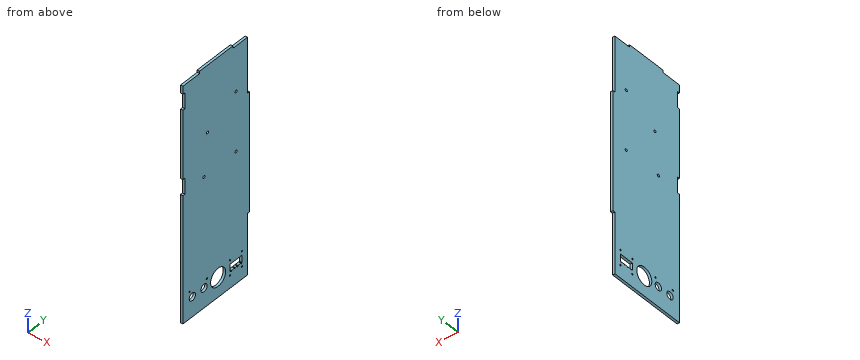
```python
from build123d import *

# Parameters (mm, degrees)
ESQUISSE1_R        = 1
ESQUISSE1_R_2      = 4.75
ESQUISSE1_R_3      = 1.6
ESQUISSE1_R_4      = 11.265
BOSS_EXTRU_1_DEPTH = 3


with BuildPart() as part:
    # Esquisse1 → Boss.-Extru.1 (new body)
    with BuildSketch(Plane(origin=(3, 0, 0), x_dir=(0, 0, -1), z_dir=(1, 0, 0))):
        Polygon((-199.626758929, -26.84585796), (-189.626758929, -26.84585796), (-189.626758929, -23.84585796), (-169.626758929, -23.84585796), (-169.626758929, -26.84585796), (-82.926758929, -26.84585796), (-82.926758929, -23.84585796), (-62.926758929, -23.84585796), (-62.926758929, -26.84585796), (97.373241071, -26.84585796), (97.373241071, 70.15414204), (20.373241071, 70.15414204), (20.373241071, 73.15414204), (-129.626758929, 73.15414204), (-129.626758929, 70.15414204), (-199.626758929, 70.15414204), (-199.626758929, 48.15414204), (-202.626758929, 48.15414204), (-202.626758929, -1.84585796), (-199.626758929, -1.84585796), align=None)
        with Locations(Location((63.373241071, -16.84585796, 0), (0, 0, 180))):
            Circle(ESQUISSE1_R, mode=Mode.SUBTRACT)
        with Locations(Location((72.373241071, 4.90414204, 0), (0, 0, 180))):
            Circle(ESQUISSE1_R_2, mode=Mode.SUBTRACT)
        with Locations(Location((-67.726758929, 53.15414204, 0), (0, 0, 180))):
            Circle(ESQUISSE1_R_3, mode=Mode.SUBTRACT)
        with Locations(Location((-118.526758929, 10.05414204, 0), (0, 0, 180))):
            Circle(ESQUISSE1_R_3, mode=Mode.SUBTRACT)
        with Locations(Location((-142.626758929, 53.15414204, 0), (0, 0, 180))):
            Circle(ESQUISSE1_R_3, mode=Mode.SUBTRACT)
        with Locations(Location((-66.426758929, 4.95414204, 0), (0, 0, 180))):
            Circle(ESQUISSE1_R_3, mode=Mode.SUBTRACT)
        with Locations(Location((72.373241071, -12.59585796, 0), (0, 0, 180))):
            Circle(ESQUISSE1_R_2, mode=Mode.SUBTRACT)
        with Locations(Location((63.373241071, 9.15414204, 0), (0, 0, 180))):
            Circle(ESQUISSE1_R, mode=Mode.SUBTRACT)
        with Locations(Location((62.423241071, 43.85414204, 0), (0, 0, 180))):
            Circle(ESQUISSE1_R, mode=Mode.SUBTRACT)
        with Locations(Location((62.423241071, 61.85414204, 0), (0, 0, 180))):
            Circle(ESQUISSE1_R, mode=Mode.SUBTRACT)
        with Locations((72.373241071, 25.996622543)):
            Circle(ESQUISSE1_R_4, mode=Mode.SUBTRACT)
        with Locations(Location((81.423241071, 43.85414204, 0), (0, 0, 180))):
            Circle(ESQUISSE1_R, mode=Mode.SUBTRACT)
        with Locations(Location((81.423241071, 61.85414204, 0), (0, 0, 180))):
            Circle(ESQUISSE1_R, mode=Mode.SUBTRACT)
        Polygon((77.423241071, 44.85414204), (76.423241071, 44.85414204), (76.423241071, 43.85414204), (67.423241071, 43.85414204), (67.423241071, 61.85414204), (76.423241071, 61.85414204), (76.423241071, 61.35414204), (77.423241071, 61.35414204), (77.423241071, 60.35414204), (76.423241071, 60.35414204), (76.423241071, 55.75414204), (77.423241071, 55.75414204), (77.423241071, 54.75414204), (76.423241071, 54.75414204), (76.423241071, 51.45414204), (77.423241071, 51.45414204), (77.423241071, 50.45414204), (76.423241071, 50.45414204), (76.423241071, 45.85414204), (77.423241071, 45.85414204), align=None, mode=Mode.SUBTRACT)
    extrude(amount=-BOSS_EXTRU_1_DEPTH)


solid = part.part
```
Here's how the part is built. I have some questions about the finished solid (model axes, mm). Give positions to 0.01 mm unless a question says otherwise; leave off trailing zeros. Order: outer loops, then holes, each group sorted by start corner. A loop starts at its lowest first (then second) coordinate and runs counter-clockwise, first axis right, second up. Notation, with made-up numbers: M 39.25,29.25 L 45.25,29.25 A33 ccw 45.25,66.25 Z; hole C -16,-8 d6. An arc over 180 degrees is marked long. Use a Markdown table: item, result. Add a question column.
1. I need wall thicknesses on probe 1 along Z at (x, y) = (0.5, 25); probe 2 along Z at (x, y) = (2.85, 55); probe 3 along Y at (x, z) = (2.2, 164.5). Which ranges of each line are inside material? Lowest first, please. Write a range as from..to.
2. Suppose I cut it at C-C (x = 2.2). Give the number of separate pieces and of enclosed holes in the cut face, and give its area (3 significant figures).
3. Suppose I cut it at A-A (y = 33). List the corners of the cut face in (x, z) for me, and give its area (3 significant figures).
4. For pin 1 Ø1.2 at (y, z) = (61.85, -81.42) entering from -X; pin 2 Ø1.1 at (x, y) = (1, 51) entering from +Z; pin 3 Ø1.5 at (x, y) = (2, 71.5) entering from -Z, each with a flat end and sliding along its axis, tell me the tip position at first contact or that it passes through.
5. Suppose I cut it at B-B (z = 163). List the corners of the cut face in (x, y) for me.
Results list:
| question | item | result |
|---|---|---|
| 1 | probe 1 | z = -97.37..-83.59, -61.15..202.63 |
| 1 | probe 2 | z = -97.37..-77.42, -67.42..199.63 |
| 1 | probe 3 | y = -26.85..70.15 |
| 2 | separate pieces | 1 |
| 2 | enclosed holes | 14 |
| 2 | area | 28,500 mm² |
| 3 | outline | M 0,-97.37 L 3,-97.37 L 3,-81.2 L 0,-81.2 Z; M 0,-63.55 L 3,-63.55 L 3,202.63 L 0,202.63 Z |
| 3 | area | 847 mm² |
| 4 | pin 1 | passes through |
| 4 | pin 2 | stops at z = 199.63 |
| 4 | pin 3 | stops at z = -20.37 |
| 5 | outline | M 0,-26.85 L 3,-26.85 L 3,70.15 L 0,70.15 Z |
